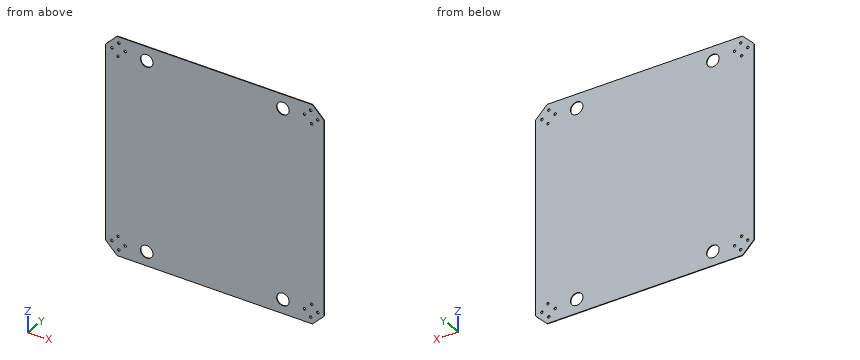
```python
from build123d import *

# Parameters (mm, degrees)
SKETCH2_R           = 2
SKETCH2_R_2         = 10
BOSS_EXTRUDE3_DEPTH = 1


with BuildPart() as part:
    # Sketch2 → Boss-Extrude3 (new body)
    with BuildSketch(Plane(origin=(0, 0, 0), x_dir=(1, 0, 0), z_dir=(0, 1, 0))):
        Polygon((-156.615, 175), (156.615, 175), (175, 156.615), (175, -156.615), (156.615, -175), (-156.615, -175), (-175, -156.615), (-175, 156.615), align=None)
        with Locations(Location((-165.100505063, 153.786572875, 0), (0, 0, 270))):
            Circle(SKETCH2_R, mode=Mode.SUBTRACT)
        with Locations(Location((-153.786572875, 165.100505063, 0), (0, 0, 270))):
            Circle(SKETCH2_R, mode=Mode.SUBTRACT)
        with Locations(Location((-155.201010127, 143.887077939, 0), (0, 0, 270))):
            Circle(SKETCH2_R, mode=Mode.SUBTRACT)
        with Locations(Location((-143.887301628, 155.200786438, 0), (0, 0, 270))):
            Circle(SKETCH2_R, mode=Mode.SUBTRACT)
        with Locations(Location((153.786572875, 165.100505063, 0), (0, 0, 270))):
            Circle(SKETCH2_R, mode=Mode.SUBTRACT)
        with Locations(Location((165.100505063, 153.786572875, 0), (0, 0, 270))):
            Circle(SKETCH2_R, mode=Mode.SUBTRACT)
        with Locations(Location((143.887077939, 155.201010127, 0), (0, 0, 270))):
            Circle(SKETCH2_R, mode=Mode.SUBTRACT)
        with Locations(Location((155.200786438, 143.887301628, 0), (0, 0, 270))):
            Circle(SKETCH2_R, mode=Mode.SUBTRACT)
        with Locations(Location((165.100505063, -153.786572875, 0), (0, 0, 270))):
            Circle(SKETCH2_R, mode=Mode.SUBTRACT)
        with Locations(Location((153.786572875, -165.100505063, 0), (0, 0, 270))):
            Circle(SKETCH2_R, mode=Mode.SUBTRACT)
        with Locations(Location((155.201010127, -143.887077939, 0), (0, 0, 270))):
            Circle(SKETCH2_R, mode=Mode.SUBTRACT)
        with Locations(Location((143.887301628, -155.200786438, 0), (0, 0, 270))):
            Circle(SKETCH2_R, mode=Mode.SUBTRACT)
        with Locations(Location((-153.786572875, -165.100505063, 0), (0, 0, 270))):
            Circle(SKETCH2_R, mode=Mode.SUBTRACT)
        with Locations(Location((-165.100505063, -153.786572875, 0), (0, 0, 270))):
            Circle(SKETCH2_R, mode=Mode.SUBTRACT)
        with Locations(Location((-143.887077939, -155.201010127, 0), (0, 0, 270))):
            Circle(SKETCH2_R, mode=Mode.SUBTRACT)
        with Locations(Location((-155.200786438, -143.887301628, 0), (0, 0, 270))):
            Circle(SKETCH2_R, mode=Mode.SUBTRACT)
        with Locations(Location((-109.204108061, 152.372583002, 0), (0, 0, 270))):
            Circle(SKETCH2_R_2, mode=Mode.SUBTRACT)
        with Locations(Location((109.204108061, 152.372583002, 0), (0, 0, 270))):
            Circle(SKETCH2_R_2, mode=Mode.SUBTRACT)
        with Locations(Location((109.204108061, -152.372583002, 0), (0, 0, 270))):
            Circle(SKETCH2_R_2, mode=Mode.SUBTRACT)
        with Locations(Location((-109.204108061, -152.372583002, 0), (0, 0, 270))):
            Circle(SKETCH2_R_2, mode=Mode.SUBTRACT)
    extrude(amount=BOSS_EXTRUDE3_DEPTH)


solid = part.part
```
Work out the finished part from the listing and answer in its coordinate system (mm). Round coordinates to 2 decimals unless told otherwise and drop trailing zeros. Write each loop counter-clockwise with the first axis right and the second up, starting at its lowest first coordinate (ties: lowest second). Pieces come first, ordered by that corner, then holes.
1) Flat-ended cylindrical pins translate along their axes: P1, Ø3.5, axis at x = 155.2, z = 143.89, coming from the +Y side; P2, Ø6.5, axis at x = -143.89, z = 155.2, coming from the -Y side. Find the tip coordinate at first contact, or state that the pin passes through.
2) A cutting plane is placed at A-A on x = -114. Determine the outline of the cut face in (y, z).
3) A cutting plane is placed at B-B on y = 0.7. Give the number of separate pieces and of enclosed holes in the cut face, and give its area (3 significant figures).
4) Consider probe 1 along Z at (x, y) = (-144, 0.35). Determine where the line is inside the solid, lowest interval first.
Entries:
1. P1: passes through
1. P2: stops at y = 0
2. outline: (0, -175) - (1, -175) - (1, -161.15) - (0, -161.15) - close; (0, -143.6) - (1, -143.6) - (1, 143.6) - (0, 143.6) - close; (0, 161.15) - (1, 161.15) - (1, 175) - (0, 175) - close
3. separate pieces: 1
3. enclosed holes: 20
3. area: 120,000 mm2
4. probe 1: z = -175 to -157.2, -153.2 to 153.2, 157.2 to 175
